Geometry check sheet. Reference: the model listing, model coordinates, mm. Face numbers are marked on the shaded views. Round coordinates to 2 decimals unless told otherwise and drop trailing zeros. Order: outer loops, then holes, each group sorted by start corner. A loop starts at its lowest first (then second) coordinate and runs counter-clockwise, first axis right, second up. Notation, with made-up numbers: (3, -23.75) - (39, -23.75) arc R30 ccw to (39, 7.25) - close; hole circle Ø9 at (59, 57). An arc over 180 degrees is marked (long way). Write each question's results on one line, items separated by ' | '.
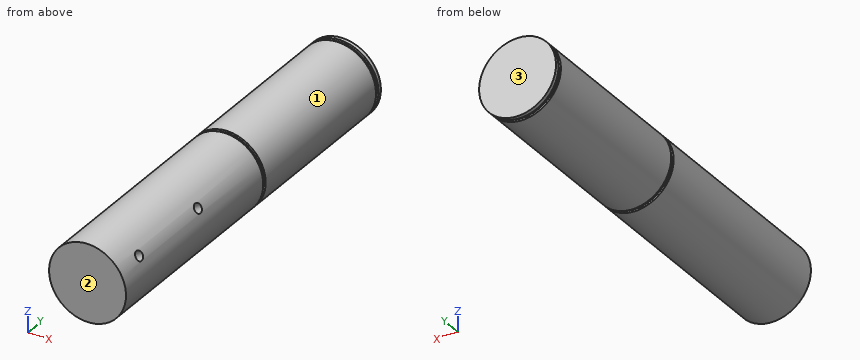
```python
from build123d import *

# Parameters (mm, degrees)
SKETCH_1_R        = 9.975
EXTRUDE_1_DEPTH   = 40
SKETCH_5_R        = 9.975
F_16MM_DEPTH      = 16
SKETCH_6_R        = 9.45
EXTRUDE_1_2_DEPTH = 1
SKETCH_7_R        = 9.975
EXTRUDE_4_DEPTH   = 45
SKETCH_8_R        = 9.45
EXTRUDE_2_DEPTH   = 1
SKETCH_9_R        = 9.975
EXTRUDE_6_DEPTH   = 1


with BuildPart() as part:
    # 草图1 → Extrude 1 (new body)
    with BuildSketch(Plane(origin=(0, 0, 0), x_dir=(1, 0, 0), z_dir=(0, 1, 0))):
        with Locations(Location((5.9, 0, 0), (0, 0, 270))):
            Circle(SKETCH_1_R)
    extrude(amount=EXTRUDE_1_DEPTH)

    # 草图4 → M3 螺纹孔2 (revolve, cut)
    with BuildSketch(Plane(origin=(14.191283323, 8, 5.545741236), x_dir=(0.555964033642643, 0, -0.8312063482047055), z_dir=(0, 1, 0))):
        Polygon((0, 0), (0, 9.251075774), (1.25, 8.5), (1.25, 0), align=None)
    hole_wizard_m3_2 = revolve(axis=Axis((19.469443634, 8, 9.076112849), (-0.8312063482047054, 0, -0.555964033642643)), mode=Mode.SUBTRACT)

    # Mirror 1364: M3 螺纹孔2 across plane
    add(hole_wizard_m3_2.mirror(Plane(origin=(0, 20, 0), x_dir=(0, 0, 1), z_dir=(0, -1, 0))), mode=Mode.SUBTRACT)

    # 草图5 → 16mm 铰链间距 (add)
    with BuildSketch(Plane(origin=(0, 40, 0), x_dir=(1, 0, 0), z_dir=(0, 1, 0))):
        with Locations(Location((5.9, 0, 0), (0, 0, 270))):
            Circle(SKETCH_5_R)
    extrude(amount=F_16MM_DEPTH)

    # 草图6 → Extrude 1 2 (add)
    with BuildSketch(Plane(origin=(0, 56, 0), x_dir=(1, 0, 0), z_dir=(0, 1, 0))):
        with Locations(Location((5.9, 0, 0), (0, 0, 270))):
            Circle(SKETCH_6_R)
    extrude(amount=EXTRUDE_1_2_DEPTH)

    # 草图7 → 凸台-拉伸4 (add)
    with BuildSketch(Plane(origin=(0, 57, 0), x_dir=(1, 0, 0), z_dir=(0, 1, 0))):
        with Locations(Location((5.9, 0, 0), (0, 0, 270))):
            Circle(SKETCH_7_R)
    extrude(amount=EXTRUDE_4_DEPTH)

    # 草图8 → 卡簧2 (add)
    with BuildSketch(Plane(origin=(0, 102, 0), x_dir=(1, 0, 0), z_dir=(0, 1, 0))):
        with Locations(Location((5.9, 0, 0), (0, 0, 270))):
            Circle(SKETCH_8_R)
    extrude(amount=EXTRUDE_2_DEPTH)

    # 草图9 → 凸台-拉伸6 (add)
    with BuildSketch(Plane(origin=(0, 103, 0), x_dir=(1, 0, 0), z_dir=(0, 1, 0))):
        with Locations(Location((5.9, 0, 0), (0, 0, 270))):
            Circle(SKETCH_9_R)
    extrude(amount=EXTRUDE_6_DEPTH)


solid = part.part
```
(1) Material ranges on line 1 (Y direction, x = 15.25, z = 3); line 2 (Y direction, x = 9.5, z = 2); line 3 (Z direction, x = 5.25, y = 67), recorded low to high.
Answers follow:
line 1: 0 to 56, 57 to 102, 103 to 104 | line 2: 0 to 6.8, 9.2 to 30.8, 33.2 to 104 | line 3: -9.95 to 9.95
(2) Section check A-A (z = -6.75). Record the cut outline in (x, y), then the cut area to 3 significant figures.
Answers follow:
outline: (-1.44, 0) - (13.24, 0) - (13.24, 56) - (12.51, 56) - (12.51, 57) - (13.24, 57) - (13.24, 102) - (12.51, 102) - (12.51, 103) - (13.24, 103) - (13.24, 104) - (-1.44, 104) - (-1.44, 103) - (-0.71, 103) - (-0.71, 102) - (-1.44, 102) - (-1.44, 57) - (-0.71, 57) - (-0.71, 56) - (-1.44, 56) - close | area: 1,520 mm²
(3) Section check B-B (y = 94). Record the cut outline in (x, z) (3 decimals).
Answers follow:
outline: circle Ø19.95 at (5.9, 0)
(4) Depth check by flat-ended pin: pin 1 Ø3 at (x, y) = (1, 12) entering from -Z; pin 2 Ø6 at (x, y) = (12, 23.5) entering from +Z; pin 3 Ø2 at (x, y) = (-0.5, 89.5) entering from -Z. Enter the tip coordinate at first touch or a pass-through.
Answers follow:
pin 1: z = -9.38 | pin 2: z = 9.48 | pin 3: z = -8.39
(5) Draft check along Y on the marked faces 1, 2 and 3. Enter one of: released by +Y, released by -Y, zero draft, split by the parting line, or undercut.
Answers follow:
face 1: zero draft | face 2: released by -Y | face 3: released by +Y
(6) Section check C-C (x = 9). Give the number of separate pieces and of enclosed holes in the cut face, then the cut area to 3 significant figures.
Answers follow:
separate pieces: 1 | enclosed holes: 2 | area: 1,960 mm²
